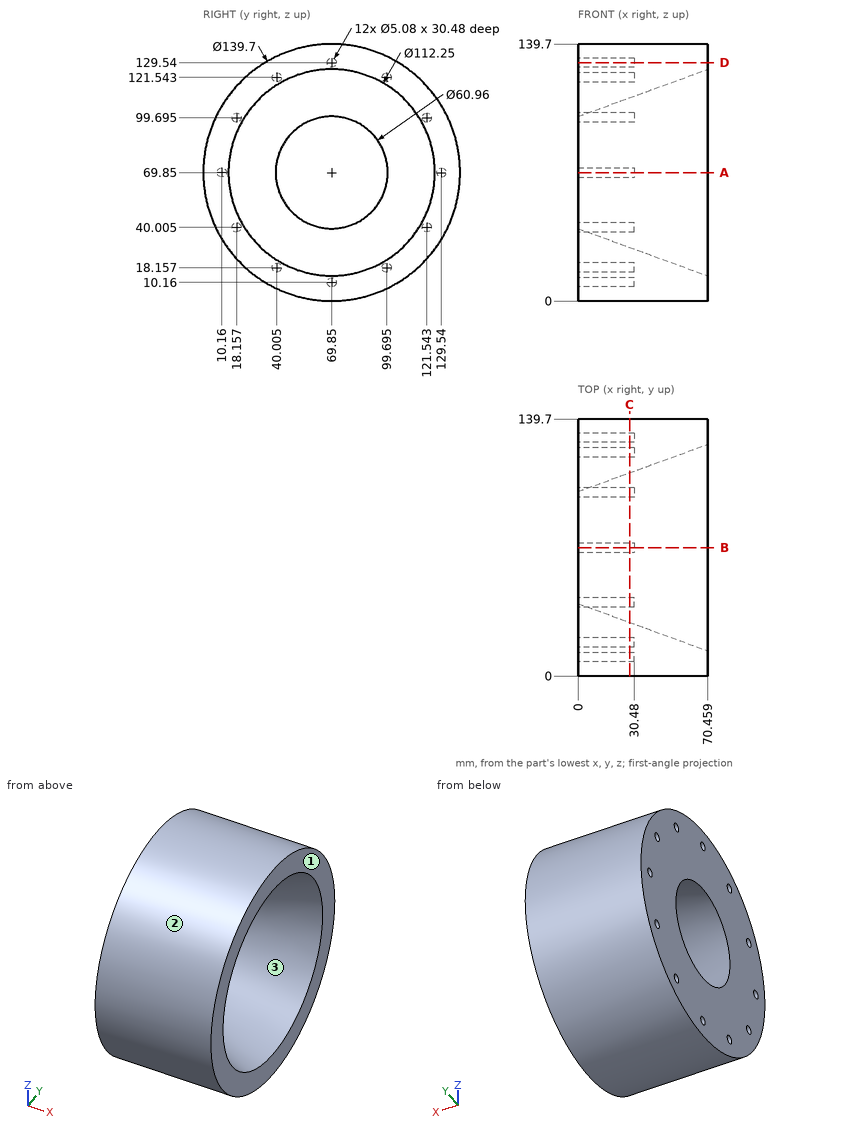
Part print with two shaded views. Sizes in mm from the minimum x, y, z corner. Coordinates: 2 decimals unless noted, no trailing zeros. Order: outer loops, then holes, each group sorted by start corner. A loop starts at its lowest first (then second) coordinate and runs counter-clockwise, first axis right, second up. Notation, with made-up numbers: M -26,26.25 L -5,26.25 A17 ccw -5,34.25 Z; hole C -11,-2.75 d7. An arc over 180 degrees is marked long. One line per question, with ' | ' between items. Start each with the question number.
1. Mould opens along Y. For the marked faces 1, 2 and 3 say: +Y half, -Y half, draft (parallel to the pull), parting line (faces both ways), or undercut.
2. Wall check: line 1 along Y through (x, z) = (59, 60); line 2 along Z through (x, y) = (11, 84); line 3 along Y through (x, z) = (13.5, 60.5) (1 decimal). Give the ranges that are in metal, low to high. Write a range as [from, to].
3. Cut at C-C (x = 28). Count the separate pieces of the cut face and the enclosed holes in it, plus the area to 3 significant figures.
4. Flat gauge pins, fed straight in: P1, Ø1.5, axis at y = 70.5, z = 10, coming from the -X side; P2, Ø3, axis at x = 7.5, z = 32, coming from the +Y side; P3, Ø2, axis at x = 48, z = 16, coming from the -Y side. Where does each tip first touch, or does it go through?
5. Cut at A-A (z = 69.85). Write the cut outline in (x, y) (1 decimal).
6. Cut at D-D (z = 129.54). Write the cut outline in (x, y).
The answers:
1) face 1: draft | face 2: parting line | face 3: undercut
2) line 1: y = [0.7, 18.84], [120.86, 139] | line 2: z = [1.45, 38.4], [101.3, 138.25] | line 3: y = [0.6, 35.7], [104, 139.1]
3) separate pieces: 1 | enclosed holes: 13 | area: 9,890 mm2
4) P1: stops at x = 30.48 | P2: stops at y = 129.5 | P3: stops at y = 24.18
5) outline: M 0,0 L 70.5,0 L 70.5,13.7 L 0,39.4 L 0,12.7 L 30.5,12.7 L 30.5,7.6 L 0,7.6 Z; M 0,100.3 L 70.5,126 L 70.5,139.7 L 0,139.7 L 0,132.1 L 30.5,132.1 L 30.5,127 L 0,127 Z
6) outline: M 0,33.57 L 70.46,33.57 L 70.46,106.13 L 0,106.13 L 0,72.39 L 30.48,72.39 L 30.48,67.31 L 0,67.31 Z
